from build123d import *

# Parameters (mm, degrees)
SKETCH1_W             = 101.6
SKETCH1_H             = 76.2
BOSS_EXTRUDE1_DEPTH   = 1.600000102
F_4_CLEARANCE_HOLE1_D = 3.4544
CHAMFER1_SIZE         = 12.7


with BuildPart() as part:
    # Sketch1 → Boss-Extrude1 (new body)
    with BuildSketch(Plane(origin=(0, 0, 0), x_dir=(1, 0, 0), z_dir=(0, 1, 0))):
        Rectangle(SKETCH1_W, SKETCH1_H)
    extrude(amount=BOSS_EXTRUDE1_DEPTH)

    # #4 Clearance Hole1 (through all)
    with Locations(Plane(origin=(0, 1.600000102, 0), x_dir=(1, 0, 0), z_dir=(0, 1, 0))):
        with Locations((38.1, -27.94), (-38.1, -27.94), (0, -27.94), (38.1, 27.94), (0, 27.94), (-38.1, 27.94)):
            Hole(F_4_CLEARANCE_HOLE1_D / 2)

    # Chamfer1
    chamfer1_edges = [part.edges().sort_by_distance(p)[0] for p in [
        (-50.8, 0.800000051, -38.1),
        (50.8, 0.800000051, -38.1),
        (50.8, 0.800000051, 38.1),
        (-50.8, 0.800000051, 38.1),
    ]]
    chamfer(chamfer1_edges, length=CHAMFER1_SIZE)


solid = part.part
Design review of the part built by this model. Coordinates are the model's own, in mm. Round coordinates to 2 decimals unless told otherwise and drop trailing zeros. Write each loop counter-clockwise with the first axis right and the second up, starting at its lowest first coordinate (ties: lowest second). Pieces come first, ordered by that corner, then holes.
Item 1: Consider section D-D on z = 32.5. Give the boundary of the cut face in (x, y).
Item 2: Consider section A-A on z = -27.94. Give the boundary of the cut face in (x, y), and give its area (3 significant figures).
Item 3: Draft analysis for pull direction Z (two halves, no side actions). For faces 1 (the cylindrical face through (-39.747, 0.789, 27.421)), 2 (the flat face through (-1, 0, -1)), 3 (the flat face through (44.5, 0.8, 31.7)), state which applies: released by +Z, released by -Z, zero draft, split by the parting line, or undercut.
Item 4: Wall thickness on L1, parallel to Z at x = 0, y = 0.55; L2, parallel to Z at x = -41, y = 1.05: over which ranges is each line inside the solid? List them lowest first.
Item 5: Consider section C-C on x = -44.5. Give the boundary of the cut face in (y, z), and give its area (3 significant figures).
Item 6: For pin 1 Ø3 at (x, z) = (0, 27.94) entering from -Y, flat-tipped, find the tip position at first contact; note if it passes through.
Item 7: Consider section B-B on y = 0.6. Give the boundary of the cut face in (x, z), and give its area (3 significant figures).
Check values:
1. outline: (-43.7, 0) - (43.7, 0) - (43.7, 1.6) - (-43.7, 1.6) - close
2. outline: (-48.26, 0) - (-39.83, 0) - (-39.83, 1.6) - (-48.26, 1.6) - close; (-36.37, 0) - (-1.73, 0) - (-1.73, 1.6) - (-36.37, 1.6) - close; (1.73, 0) - (36.37, 0) - (36.37, 1.6) - (1.73, 1.6) - close; (39.83, 0) - (48.26, 0) - (48.26, 1.6) - (39.83, 1.6) - close
2. area: 138 mm2
3. face 1: undercut
3. face 2: zero draft
3. face 3: released by +Z
4. L1: z = -38.1 to -29.67, -26.21 to 26.21, 29.67 to 38.1
4. L2: z = -35.2 to 35.2
5. outline: (0, -31.7) - (1.6, -31.7) - (1.6, 31.7) - (0, 31.7) - close
5. area: 101 mm2
6. pin 1: passes through
7. outline: (-50.8, -25.4) - (-38.1, -38.1) - (38.1, -38.1) - (50.8, -25.4) - (50.8, 25.4) - (38.1, 38.1) - (-38.1, 38.1) - (-50.8, 25.4) - close; hole circle Ø3.45 at (-38.1, -27.94); hole circle Ø3.45 at (-38.1, 27.94); hole circle Ø3.45 at (0, -27.94); hole circle Ø3.45 at (0, 27.94); hole circle Ø3.45 at (38.1, -27.94); hole circle Ø3.45 at (38.1, 27.94)
7. area: 7,360 mm2
